Source: CAD feature listing. Evaluate the final solid. Frame: model axes, mm. A direction names the side the tool comes from. Coordinates: 2 decimals unless noted, no trailing zeros. Order: outer loops, then holes, each group sorted by start corner. A loop starts at its lowest first (then second) coordinate and runs counter-clockwise, first axis right, second up.
```python
from build123d import *

# Parameters (mm, degrees)
F1_DEPTH = 76.2
F2_W     = 29.3097225949
F2_H     = 14.7436801344
F3_DEPTH = 76.2
F5_DEPTH = 31.8535955081
F6_R     = 5.08


with BuildPart() as f1:
    # F0 (on Front) → F1 (new body)
    with BuildSketch(Plane.XZ):
        Polygon((-39.5237128198, -19.4368070878), (-39.5237128198, -44.8368070878), (36.6762871802, -44.8368070878), (36.6762871802, -19.4368070878), (11.2762871802, -19.4368070878), (11.2762871802, 44.0631929122), (36.6762871802, 44.0631929122), (36.6762871802, 67.8244820096), (-39.5237128198, 67.8244820096), (-39.5237128198, 44.0631929122), (-14.1237131261, 44.0631929122), (-14.1237131261, -19.4368070878), align=None)
    extrude(amount=F1_DEPTH)

    # F2 (on face) → F3 (join)
    with BuildSketch(Plane.XY.offset(67.8244820096)):
        with Locations((-19.8845365085, -24.4807554409)):
            Rectangle(F2_W, F2_H)
    extrude(amount=F3_DEPTH)

    # F4 (on face) → F5 (cut, through all)
    with BuildSketch(Plane.XZ.offset(31.8525955081)):
        Polygon((-17.5263217899, 115.0952721356), (-28.6504694012, 112.3630260708), (-31.8463487054, 101.3631086114), (-23.9180803982, 93.0954372169), (-12.7939327868, 95.8276832817), (-9.5980534826, 106.8276007411), align=None)
    extrude(amount=-F5_DEPTH, mode=Mode.SUBTRACT)

    # F6
    f6_edges = [f1.edges().sort_by_distance(p)[0] for p in [
        (-1.423713, -76.2, 67.824482),
        (36.676287, -38.1, 67.824482),
        (36.676287, -38.1, 44.063193),
        (36.676287, 0, 55.943837),
        (36.676287, -76.2, 55.943837),
        (-26.823713, -76.2, 44.063193),
        (-14.123713, -76.2, 12.313193),
        (-26.823713, -76.2, -19.436807),
        (-39.523713, -76.2, -32.136807),
        (-1.423713, -76.2, -44.836807),
        (36.676287, -76.2, -32.136807),
        (23.976287, -76.2, -19.436807),
        (11.276287, -76.2, 12.313193),
        (23.976287, -76.2, 44.063193),
        (-39.523713, -76.2, 55.943837),
    ]]
    fillet(f6_edges, radius=F6_R)


solid = f1.part
```
1. Section query C-C on z = 39. Return loops of the section in (x, y).
Findings:
outline: (-14.12, -71.12) arc R5.08 ccw to (-9.04, -76.2) - (6.2, -76.2) arc R5.08 ccw to (11.28, -71.12) - (11.28, 0) - (-14.12, 0) - close
2. Pin query (flat end, axial travel): P1, Ø7.5, axis at y = -27, z = 106.5, coming from the -X side; P2, Ø3, axis at x = -30.5, z = 104, coming from the -Y side; P3, Ø12, axis at y = -22.5, z = 105, coming from the +X side. Return the tip coordinate at first contact, or that it passes through.
Findings:
P1: stops at x = -34.54
P2: stops at y = -31.85
P3: stops at x = -5.23
3. Access query for faces 4 (the face through (-12.6, -74.75, 11.8)), 5 (the face through (24, -35, -19.437)), 6 (the face through (-27, -35, -19.437)), 7 (the face through (-23.01, -24.58, 113.75)). Directions: +Z, -Z, +X, -X, +Y, -Y. A direction counts if a zero-diameter tool reaches every point of the face in a straight line with its end or side. Return the directions, or none.
Findings:
face 4: -X, -Y
face 5: +X, +Y, -Y
face 6: -X, +Y, -Y
face 7: +Y, -Y
4. Ray query, line 1 (Z direction, x = -20.5, y = -5.5); line 2 (Z direction, x = -1.5, y = -70.5); line 3 (X direction, y = -60, z = -16). Return the intervals inside material, ascending.
Findings:
line 1: z = -44.84 to -19.44, 44.06 to 67.82
line 2: z = -44.84 to 67.82
line 3: x = -14.12 to 11.28
5. Section query B-B on x = -1. Return loops of the section in (y, z), plus the area to 3 significant figures.
Findings:
outline: (-76.2, -39.76) arc R5.08 ccw to (-71.12, -44.84) - (0, -44.84) - (0, 67.82) - (-71.12, 67.82) arc R5.08 ccw to (-76.2, 62.74) - close
area: 8,570 mm2
6. Section query D-D on y = -53. Return loops of the section in (x, z).
Findings:
outline: (-39.52, -44.84) - (36.68, -44.84) - (36.68, -19.44) - (11.28, -19.44) - (11.28, 44.06) - (31.6, 44.06) arc R5.08 ccw to (36.68, 49.14) - (36.68, 62.74) arc R5.08 ccw to (31.6, 67.82) - (-39.52, 67.82) - (-39.52, 44.06) - (-14.12, 44.06) - (-14.12, -19.44) - (-39.52, -19.44) - close
7. Section query A-A on y = -19. Return loops of the section in (x, z).
Findings:
outline: (-39.52, -44.84) - (36.68, -44.84) - (36.68, -19.44) - (11.28, -19.44) - (11.28, 44.06) - (31.6, 44.06) arc R5.08 ccw to (36.68, 49.14) - (36.68, 62.74) arc R5.08 ccw to (31.6, 67.82) - (-5.23, 67.82) - (-5.23, 144.02) - (-34.54, 144.02) - (-34.54, 67.82) - (-39.52, 67.82) - (-39.52, 44.06) - (-14.12, 44.06) - (-14.12, -19.44) - (-39.52, -19.44) - close; hole (-31.85, 101.36) - (-23.92, 93.1) - (-12.79, 95.83) - (-9.6, 106.83) - (-17.53, 115.1) - (-28.65, 112.36) - close
8. Draft query along X for faces 1 (the face through (-30.226, -24.584, 106.94)), 2 (the face through (-27, -35, 44.063)), 3 (the face through (9.7, -74.8, 12.8)). Return one class per face: released by +X, released by -X, zero draft, split by the parting line, or undercut.
Findings:
face 1: undercut
face 2: zero draft
face 3: released by +X
